from build123d import *

# Parameters (mm, degrees)
SKETCH1_R           = 21.25
BOSS_EXTRUDE1_DEPTH = 2
SKETCH2_R           = 11.75
BOSS_EXTRUDE2_DEPTH = 1.5
FILLET1_R           = 0.5
CUT_EXTRUDE2_DEPTH  = 4.5
SKETCH5_R           = 1.654382936
CUT_EXTRUDE3_DEPTH  = 0.01
CIRPATTERN1_COUNT   = 8


with BuildPart() as part:
    # Sketch1 → Boss-Extrude1 (new body)
    with BuildSketch(Plane(origin=(0, 0, 0), x_dir=(1, 0, 0), z_dir=(0, 1, 0))):
        Circle(SKETCH1_R)
    extrude(amount=BOSS_EXTRUDE1_DEPTH)

    # Sketch2 → Boss-Extrude2 (add)
    with BuildSketch(Plane(origin=(0, 2, 0), x_dir=(1, 0, 0), z_dir=(0, 1, 0))):
        Circle(SKETCH2_R)
    extrude(amount=BOSS_EXTRUDE2_DEPTH)

    # Fillet1
    fillet1_edges = [part.edges().sort_by_distance(p)[0] for p in [
        (-11.75, 3.5, 0),
    ]]
    fillet(fillet1_edges, radius=FILLET1_R)

    # Sketch4 → Cut-Extrude2 (cut, through all)
    with BuildSketch(Plane.XZ):
        with BuildLine():
            Line((-2.5, 19.54), (-2.5, 23.75))
            Line((-2.5, 23.75), (2.5, 23.75))
            Line((2.5, 23.75), (2.5, 19.54))
            ThreePointArc((2.5, 19.54), (0, 17.04), (-2.5, 19.54))
        make_face()
    cut_extrude2 = extrude(amount=-CUT_EXTRUDE2_DEPTH, mode=Mode.SUBTRACT)

    # Sketch5 → Cut-Extrude3 (cut)
    with BuildSketch(Plane(origin=(0, 0, 0), x_dir=(-1, 0, 0), z_dir=(0, -1, 0))):
        Circle(SKETCH5_R)
    extrude(amount=-CUT_EXTRUDE3_DEPTH, mode=Mode.SUBTRACT)

    # CirPattern1: Cut-Extrude2 ×8 about axis
    cirpattern1_axis = Axis((0, 0, 0), (0, 1, 0))
    for i in range(1, CIRPATTERN1_COUNT):
        add(cut_extrude2.rotate(cirpattern1_axis, i * 360 / CIRPATTERN1_COUNT), mode=Mode.SUBTRACT)


solid = part.part
Source: CAD feature listing. Evaluate the final solid. Frame: model axes, mm. A direction names the side the tool comes from. Coordinates: 2 decimals unless noted, no trailing zeros. Order: outer loops, then holes, each group sorted by start corner. A loop starts at its lowest first (then second) coordinate and runs counter-clockwise, first axis right, second up.
Item 1: Cut plane D-D (x = -15). Return loops of the section in (y, z).
Output values:
outline: (0, -11.61) - (2, -11.61) - (2, 11.61) - (0, 11.61) - close
Item 2: First-contact query: P1, Ø0.8, axis at y = 1, z = -20, coming from the +X side; P2, Ø1.7, axis at x = 20, y = 0.5, coming from the -Z side; P3, Ø2, axis at x = -4, y = 1, coming from the -Z side. Flat tips, straight axial feed; report the tip coordinate or a pass-through.
Output values:
P1: stops at x = 8.21
P2: stops at z = -9.21
P3: stops at z = -21.04
Item 3: Set-up query: faces 4 (the face through (-12.609, 0.986, 16.145)), 5 (the face through (11.207, 2.493, -3.529)), 6 (the face through (-2.5, 1, -20)). Return all of +Z, -Z, +X, -X, +Y, -Y with unobstructed straight access to the full face (end or side cutting, diameter ignored); none if empty.
Output values:
face 4: -X, +Y, -Y
face 5: +Y
face 6: -Z, +Y, -Y
Item 4: Material intervals for line 1 (X direction, y = 1.8, z = -12.5); line 2 (Y direction, x = -16.5, z = 5); line 3 (Z direction, x = 0, y = 0.05), sorted ascending.
Output values:
line 1: x = -17.18 to -16.04, -11.69 to 11.69, 16.04 to 17.18
line 2: y = 0 to 2
line 3: z = -17.04 to 17.04
Item 5: Pull-direction query (Z, two-part tool) for faces 1 (the face through (-19.6, 0.99, -8.21)), 2 (the face through (-12.594, 0.986, -16.129)), 3 (the face through (4, 0, 0)); classes: pulls with the +Z half, pulls with the -Z half, needs draft (parallel to the pull), parting line crosses it, or undercut.
Output values:
face 1: pulls with the -Z half
face 2: undercut
face 3: needs draft
